Verification items for the finished model (mm, model axes). A direction names the side the tool comes from. Coordinates: 2 decimals unless noted, no trailing zeros. Loops run counter-clockwise (first coordinate to the right, second up) from the corner with the lowest first, then second, coordinate; pieces in that order, holes last. Notation, with made-up numbers: (-37, 60.25) - (-18, 60.25) arc R35 ccw to (-18, 99.25) - close; hole circle Ø11 at (-4, -37.75). An arc over 180 degrees is marked (long way). Answer as CSV lines item,"result". Start each with the question number.
1. Material ranges on line 1 (Y direction, x = 0, z = 50.75); line 2 (Z direction, x = -0.5, y = -1.75); line 3 (X direction, y = -0.25, z = 35), recorded low to high. Write a range as [from, to].
2. Cross-section at D-D (y = -5). Enter the section's corners in (x, z).
3. Cross-section at B-B (y = 0). Enter the section's corners in (x, z), plus the area to 3 significant figures.
4. Cross-section at A-A (x = 0). Enter the section's corners in (y, z).
5. Gauge pin test, flat ends, axial feed: P1, Ø2.5, axis at x = 0, y = -0.5, coming from the +Z side; P2, Ø1.5, axis at y = -3.5, z = 44.5, coming from the -X side; P3, Ø3.5, axis at y = -0.5, z = 27, coming from the +X side. Record the tip position at first contact, or that the pin passes through.
6. Release check for a two-part mould opening along X. For faces 1 (the flat face through (0, 0, 41)), 2 (the flat face through (-5.4, 0, 33)), 3 (the cylindrical face through (-4.76, 3.65, 26.13)) record: pulls with the +X half, pulls with the -X half, needs draft (parallel to the pull), parting line crosses it, or undercut.
7. Cross-section at C-C (z = 19.5). Enter the section's corners in (x, y), plus the area to 3 significant figures.
8. Set-up check for faces 4 (the flat face through (5, 0, 28)), 5 (the cylindrical face through (0.54, 2.44, 47.08)), 6 (the flat face through (-5.4, 0, 23)): record each of +Z, -Z, +X, -X, +Y, -Y from which the full face is reachable in a straight line by a thin tool's end or side.
Autodesk Fusion 360 part; units mm, degrees
sketch "Esquisse1" plane through (0, 0, 0) normal (0, 0, 1) x (1, 0, 0)
  circle A0 centre (0, 0) radius 6
  dimension "d1" = 12
extrude "Extrusion1" add sketch "Esquisse1" along normal blind 53
sketch "Esquisse2" plane through (0, 0, 53) normal (0, 0, 1) x (-1, 0, 0)
  circle A0 centre (0, 0) radius 6
  circle A1 centre (0, 0) radius 2.5
  dimension "d5" = 5
extrude "Extrusion2" cut sketch "Esquisse2" against normal blind 12 contours A1
sketch "Esquisse3" plane through (0, 0, 0) normal (0, 0, -1) x (1, 0, 0)
  circle A0 centre (0, 0) radius 6
  circle A1 centre (0, 0) radius 2.5
  dimension "d8" = 5
extrude "Extrusion3" cut sketch "Esquisse3" against normal blind 12 contours A1
sketch "Esquisse4" plane through (0, 0, 53) normal (0, 0, 1) x (-1, 0, 0)
  circle A0 centre (0, 0) radius 2.5
  circle A1 centre (0, 0) radius 6
  line L0 (5, 8) -> (-5, 8)
  line L1 (-5, 8) -> (-5, -7.4606)
  line L2 (-5, -7.4606) -> (5, -7.4606)
  line L3 (5, -7.4606) -> (5, 8)
  dimension "d11" = 5
  dimension "d12" = 10
extrude "Extrusion4" cut sketch "Esquisse4" against normal blind 10 from surface at -20 contours A1 L3 | A1 L1
Values follow:
1,line 1,"y = [-6, -2.5], [2.5, 6]"
1,line 2,"z = [12, 41]"
1,line 3,"x = [-5.99, 5.99]"
2,outline,"(-3.32, 0) - (3.32, 0) - (3.32, 53) - (-3.32, 53) - close"
3,outline,"(-6, 0) - (-2.5, 0) - (-2.5, 12) - (2.5, 12) - (2.5, 0) - (6, 0) - (6, 23) - (5, 23) - (5, 33) - (6, 33) - (6, 53) - (2.5, 53) - (2.5, 41) - (-2.5, 41) - (-2.5, 53) - (-6, 53) - (-6, 33) - (-5, 33) - (-5, 23) - (-6, 23) - close"
3,area,"496 mm²"
4,outline,"(-6, 0) - (-2.5, 0) - (-2.5, 12) - (2.5, 12) - (2.5, 0) - (6, 0) - (6, 53) - (2.5, 53) - (2.5, 41) - (-2.5, 41) - (-2.5, 53) - (-6, 53) - close"
5,P1,"stops at z = 41"
5,P2,"stops at x = -5.33"
5,P3,"stops at x = 5"
6,face 1,"undercut"
6,face 2,"needs draft"
6,face 3,"parting line crosses it"
7,outline,"circle Ø12 at (0, 0)"
7,area,"113 mm²"
8,face 4,"+X, +Y, -Y"
8,face 5,"+Z"
8,face 6,"-X, +Y, -Y"
